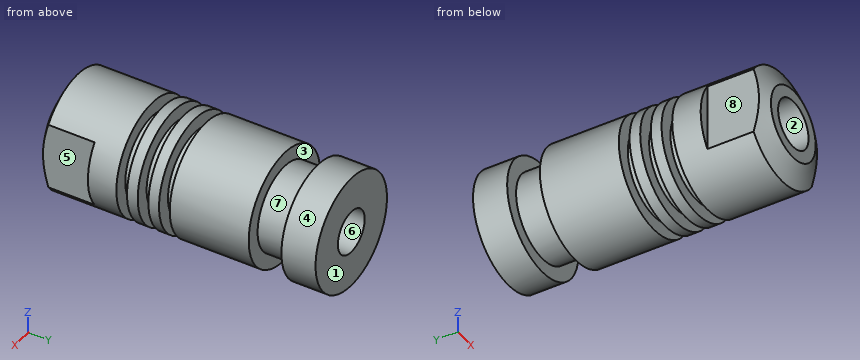
```python
from build123d import *

# Parameters (mm, degrees)
TAGLIO_ESTRUSIONE1_REACH             = 10
SCHIZZO2_W                           = 1.5
SCHIZZO2_H                           = 8
TAGLIO_ESTRUSIONE1_DIRECTION_2_REACH = 10
SCHIZZO7_R                           = 3
TAGLIO_ESTRUSIONE2_DEPTH             = 41
FORO_FILETTATO_M8_1_D                = 6.8
FORO_FILETTATO_M8_1_DEPTH            = 12
FORO_FILETTATO_M8_1_TIP              = 2.042926105


with BuildPart() as part:
    # Schizzo1 → Rivoluzione1 (revolve)
    with BuildSketch(Plane.XY):
        Polygon((0, 0), (-5, 0), (-8, 1.5), (-8, 12), (-6, 12), (-6, 13.5), (-8, 13.5), (-8, 15), (-6, 15), (-6, 16.5), (-8, 16.5), (-8, 18), (-6, 18), (-6, 19.5), (-8, 19.5), (-8, 30.6), (-6, 30.6), (-6, 35.2), (-8, 35.2), (-8, 40), (0, 40), align=None)
    revolve(axis=Axis((0, 129.407380346, 0), (0, -1, 0)))

    # Schizzo2 → Taglio-Estrusione1 (cut, up to next)
    with BuildSketch(Plane.XY, mode=Mode.PRIVATE) as taglio_estrusione1_sk1:
        with Locations((-7.25, 4)):
            Rectangle(SCHIZZO2_W, SCHIZZO2_H)
    taglio_estrusione1_tool1 = extrude(taglio_estrusione1_sk1.sketch, amount=-TAGLIO_ESTRUSIONE1_REACH, mode=Mode.PRIVATE) & part.part
    add(taglio_estrusione1_tool1.solids().sort_by_distance((-7.25, 4, 0))[0], mode=Mode.SUBTRACT)
    # Schizzo2 → Taglio-Estrusione1 (cut, up to next)
    with BuildSketch(Plane.XY, mode=Mode.PRIVATE) as taglio_estrusione1_sk2:
        with Locations((7.25, 4)):
            Rectangle(SCHIZZO2_W, SCHIZZO2_H)
    taglio_estrusione1_tool2 = extrude(taglio_estrusione1_sk2.sketch, amount=-TAGLIO_ESTRUSIONE1_REACH, mode=Mode.PRIVATE) & part.part
    add(taglio_estrusione1_tool2.solids().sort_by_distance((7.25, 4, 0))[0], mode=Mode.SUBTRACT)

    # Schizzo2 → Taglio-Estrusione1 direction 2 (cut, up to next)
    with BuildSketch(Plane.XY, mode=Mode.PRIVATE) as taglio_estrusione1_direction_2_sk1:
        with Locations((-7.25, 4)):
            Rectangle(SCHIZZO2_W, SCHIZZO2_H)
    taglio_estrusione1_direction_2_tool1 = extrude(taglio_estrusione1_direction_2_sk1.sketch, amount=TAGLIO_ESTRUSIONE1_DIRECTION_2_REACH, mode=Mode.PRIVATE) & part.part
    add(taglio_estrusione1_direction_2_tool1.solids().sort_by_distance((-7.25, 4, 0))[0], mode=Mode.SUBTRACT)
    # Schizzo2 → Taglio-Estrusione1 direction 2 (cut, up to next)
    with BuildSketch(Plane.XY, mode=Mode.PRIVATE) as taglio_estrusione1_direction_2_sk2:
        with Locations((7.25, 4)):
            Rectangle(SCHIZZO2_W, SCHIZZO2_H)
    taglio_estrusione1_direction_2_tool2 = extrude(taglio_estrusione1_direction_2_sk2.sketch, amount=TAGLIO_ESTRUSIONE1_DIRECTION_2_REACH, mode=Mode.PRIVATE) & part.part
    add(taglio_estrusione1_direction_2_tool2.solids().sort_by_distance((7.25, 4, 0))[0], mode=Mode.SUBTRACT)

    # Schizzo7 → Taglio-Estrusione2 (cut, through all)
    with BuildSketch(Plane(origin=(0, 40, 0), x_dir=(1, 0, 0), z_dir=(0, 1, 0))):
        Circle(SCHIZZO7_R)
    extrude(amount=-TAGLIO_ESTRUSIONE2_DEPTH, mode=Mode.SUBTRACT)

    # Foro filettato M8-1
    with Locations(Plane(origin=(0, 0, 0), x_dir=(-1, 0, 0), z_dir=(0, -1, 0))):
        with Locations((0, 0)):
            Hole(FORO_FILETTATO_M8_1_D / 2, depth=FORO_FILETTATO_M8_1_DEPTH)
            with Locations((0, 0, -(FORO_FILETTATO_M8_1_DEPTH + FORO_FILETTATO_M8_1_TIP / 2))):  # 118° drill point
                Cone(0, FORO_FILETTATO_M8_1_D / 2, FORO_FILETTATO_M8_1_TIP, mode=Mode.SUBTRACT)


solid = part.part
```
Geometry check sheet. Reference: the model listing, model coordinates, mm. Face numbers are marked on the shaded views. A direction names the side the tool comes from. Give positions to 0.01 mm unless a question says otherwise; leave off trailing zeros. Order: outer loops, then holes, each group sorted by start corner. A loop starts at its lowest first (then second) coordinate and runs counter-clockwise, first axis right, second up.
1. Section check B-B, the plane y = 11. Enter the section's corners in (x, z).
2. Thickness scan on L1, parallel to X at y = 18.25, z = 0; L2, parallel to Z at x = 0, y = 9.25; L3, parallel to Z at x = 0, y = 22.5. Record the ranges inside material, lowest first.
3. Gauge pin test, flat ends, axial feed: pin 1 Ø1.5 at (x, y) = (2.5, 17) entering from -Z; pin 2 Ø1.5 at (y, z) = (28.5, 2.5) entering from -X; pin 3 Ø1.5 at (x, z) = (1, -6) entering from -Y. Record the tip position at first contact, or that the pin passes through.
4. Access from +Z, -Z, +X, -X, +Y, -Y to the whole of each face (thin tool, end or side, straight path). Record for the marked faces 1, 2, 3, 4 and 5.
5. Release check for a two-part mould opening along X. For the marked faces 6, 7 and 8 record: pulls with the +X half, pulls with the -X half, needs draft (parallel to the pull), parting line crosses it, or undercut.
6. Section check A-A, the plane y = 31. Enter the section's corners in (x, z).
Values follow:
1. outline: circle Ø16 at (0, 0); hole circle Ø6.8 at (0, 0)
2. L1: x = -6 to -3, 3 to 6
2. L2: z = -8 to -3.4, 3.4 to 8
2. L3: z = -8 to -3, 3 to 8
3. pin 1: stops at z = -7.81
3. pin 2: stops at x = -7.81
3. pin 3: stops at y = 0.17
4. face 1: +Z, -Z, +X, -X, +Y
4. face 2: -Y
4. face 3: none
4. face 4: +Y, -Y
4. face 5: +Z, -Z, +X, -Y
5. face 6: undercut
5. face 7: parting line crosses it
5. face 8: pulls with the -X half
6. outline: circle Ø12 at (0, 0); hole circle Ø6 at (0, 0)
